Autodesk Inventor part; units mm, degrees
ref_plane "YZ Plane" through (0, 0, 0) normal (1, 0, 0) x (0, 1, 0)
ref_plane "XZ Plane" through (0, 0, 0) normal (0, 1, 0) x (-1, 0, 0)
ref_plane "XY Plane" through (0, 0, 0) normal (0, 0, 1) x (1, 0, 0)
sketch "スケッチ1" plane through (0, 0, 0) normal (1, 0, 0) x (0, 1, 0)
  line L0 (0, 0) -> (0, -38)
  line L1 (0, -38) -> (-10, -38)
  line L2 (-10, -38) -> (-10, 0)
  line L3 (-10, 0) -> (0, 0)
  dimension "d0" = 38
  dimension "d2" = 10
extrude "プレート1" add sketch "スケッチ1" along normal blind 2
sketch "スケッチ14" plane through (-2, 2, -38) normal (0, 1, 0) x (-1, 0, 0)
  line L0 (0, 38) -> (0, 0)
  line L1 (0, 0) -> (8, 0)
  line L2 (8, 0) -> (8, 38)
  line L3 (8, 38) -> (0, 38)
edge flange "フランジ1" height 12 angle 90 thickness 2 bend radius 2 thickness toward (0, 1, 0) relief tear relief width 2 relief depth 1 edges at (0, 0, -19) wall of the first edge with corners at (-2, 2, 0) (-2, 2, -38) (-10, 2, -38) (-10, 2, 0)
bend "曲げ26"
corner "コーナー1"
sketch "スケッチ15" plane through (-2, -12, 0) normal (0, -1, 0) x (1, 0, 0)
  line L0 (0, -38) -> (0, 0)
  line L1 (0, 0) -> (-8, 0)
  line L2 (-8, 0) -> (-8, -38)
  line L3 (-8, -38) -> (0, -38)
edge flange "フランジ2" height 12 angle 90 thickness 2 bend radius 2 thickness toward (0, -1, 0) relief tear relief width 2 relief depth 1 edges at (0, -10, -19) wall of the first edge with corners at (-2, -12, -38) (-2, -12, 0) (-10, -12, 0) (-10, -12, -38)
bend "曲げ27"
corner "コーナー2"
sketch "スケッチ16" plane through (-10, 4, 0) normal (0, 1, 0) x (1, 0, 0)
  line L0 (5.5, 4) -> (5.5, 34)
  arc A0 (5.5, 34) -> (2.5, 34) centre (4, 34) ccw
  line L1 (2.5, 34) -> (2.5, 4)
  arc A1 (2.5, 4) -> (5.5, 4) centre (4, 4) ccw
  line L2 (0, 38) -> (8, 38)
  line L3 (8, 0) -> (0, 0)
  point P0 (10, 0)
  point P1 (4, 38)
  dimension "d192" = 1.5
  dimension "d193" = 4
  dimension "d194" = 4
extrude "押し出し1" cut sketch "スケッチ16" against normal blind 10
sketch "スケッチ17" plane through (-10, -12, 0) normal (0, 1, 0) x (1, 0, 0)
  line L0 (0, 0) -> (8, 0)
  line L1 (0, 38) -> (8, 38)
  point P0 (10, 0)
  point P1 (4, 5)
  point P2 (4, 33)
  point P3 (4, 0)
  point P4 (4, 38)
  dimension "d197" = 5
  dimension "d198" = 5
hole "穴1" at (-6, -12, -5) at (-6, -12, -33) direction (0, -1, 0) diameter 3 end through all
equation "\"d204\" = Thickness"
equation "\"d3\" = Thickness"
equation "\"d172\" = BendReliefWidth"
equation "\"d173\" = BendReliefDepth"
equation "\"d174\" = MinimumRemnant"
equation "\"d175\" = TransitionRadius"
equation "\"d178\" = BendRadius"
equation "\"d179\" = CornerReliefSize"
equation "\"d180\" = GapSize"
equation "\"d181\" = JacobiRadiusSize"
equation "\"d182\" = BendReliefWidth"
equation "\"d183\" = BendReliefDepth"
equation "\"d184\" = MinimumRemnant"
equation "\"d185\" = TransitionRadius"
equation "\"d188\" = BendRadius"
equation "\"d189\" = CornerReliefSize"
equation "\"d190\" = GapSize"
equation "\"d191\" = JacobiRadiusSize"
equation "\"BendRadius\" = Thickness"
equation "\"BendReliefWidth\" = Thickness"
equation "\"BendReliefDepth\" = 0.5 * Thickness"
equation "\"CornerReliefSize\" = 4 * Thickness"
equation "\"MinimumRemnant\" = 2 * Thickness"
equation "\"TransitionRadius\" = BendRadius"
equation "\"JacobiRadiusSize\" = BendRadius"
equation "\"GapSize\" = Thickness"
properties part number "frame_front" material "アルミニウム 6061"
Geometry check sheet. Reference: the model listing, model coordinates, mm. A direction names the side the tool comes from. Round coordinates to 2 decimals unless told otherwise and drop trailing zeros. Order: outer loops, then holes, each group sorted by start corner. A loop starts at its lowest first (then second) coordinate and runs counter-clockwise, first axis right, second up. Notation, with made-up numbers: M -25,72 L -5,72 A17 ccw -5,92 Z; hole C 54,17 d5. An arc over 180 degrees is marked long. Answer in a Markdown table with one row per item.
(1) Draft check along Y on faces 4 (the face through (0.4, -5.7, 0)), 5 (the face through (0.797, -12.859, -18.734)), 6 (the face through (-8, 4, -19)), 7 (the face through (-0.6, 1.43, -19.27)). Enter one of: released by +Y, released by -Y, zero draft, split by the parting line, or undercut.
Responses:
| item | result |
|---|---|
| face 4 | zero draft |
| face 5 | released by -Y |
| face 6 | released by +Y |
| face 7 | undercut |
(2) Sectioned sample at B-B, the plane x = -6. Record the cut outline in (y, z), and give its area (3 significant figures).
Responses:
| item | result |
|---|---|
| outline | M -14,-38 L -12,-38 L -12,-34.5 L -14,-34.5 Z; M -14,-31.5 L -12,-31.5 L -12,-6.5 L -14,-6.5 Z; M -14,-3.5 L -12,-3.5 L -12,0 L -14,0 Z; M 2,-38 L 4,-38 L 4,-35.5 L 2,-35.5 Z; M 2,-2.5 L 4,-2.5 L 4,0 L 2,0 Z |
| area | 74.0 mm² |
(3) Sectioned sample at A-A, the plane x = -2.5. Record the cut outline in (y, z), and give its area (3 significant figures).
Responses:
| item | result |
|---|---|
| outline | M -14,-38 L -12,-38 L -12,0 L -14,0 Z; M 2,-38 L 4,-38 L 4,0 L 2,0 Z |
| area | 152 mm² |
(4) Sectioned sample at C-C, the plane z = -10. Record the cut outline in (x, y), and give its area (3 significant figures).
Responses:
| item | result |
|---|---|
| outline | M -10,-14 L -2,-14 A4 ccw 2,-10 L 2,0 A4 ccw -2,4 L -4.5,4 L -4.5,2 L -2,2 A2 cw 0,0 L 0,-10 A2 cw -2,-12 L -10,-12 Z; M -10,2 L -7.5,2 L -7.5,4 L -10,4 Z |
| area | 64.8 mm² |
(5) Go/stop test with flat-tipped pins: P1, Ø2.5, axis at x = -6, z = -33, coming from the -Y side; P2, Ø8, axis at y = -7, z = -18.5, coming from the -X side; P3, Ø1.6, axis at y = 3.5, z = -13.5, coming from the +X side; P4, Ø8, axis at y = -6, z = -21, coming from the -X side. Record where each tip stops, or that it passes through.
Responses:
| item | result |
|---|---|
| P1 | passes through |
| P2 | stops at x = -0.27 |
| P3 | stops at x = 0.95 |
| P4 | stops at x = 0 |
(6) Sectioned sample at D-D, the plane z = -5.5. Record the cut outline in (x, y).
Responses:
| item | result |
|---|---|
| outline | M -10,-14 L -7.41,-14 L -7.41,-12 L -10,-12 Z; M -10,2 L -7.5,2 L -7.5,4 L -10,4 Z; M -4.59,-14 L -2,-14 A4 ccw 2,-10 L 2,0 A4 ccw -2,4 L -4.5,4 L -4.5,2 L -2,2 A2 cw 0,0 L 0,-10 A2 cw -2,-12 L -4.59,-12 Z |
(7) Tool access check on faces 1 (the face through (-7.5, 3, -19)), 2 (the face through (-5.1, -13, -34.2)), 3 (the face through (-6, -12, -19)). Record the directions out of +Z, -Z, +X, -X, +Y, -Y that give a thin tool (end or side, any length) a straight path to the whole face; none if there is none.
Responses:
| item | result |
|---|---|
| face 1 | +Y |
| face 2 | +Y, -Y |
| face 3 | +Z, -Z, -X |
(8) Scan lines: probe 1 along Z at (x, y) = (-6, -13.1); probe 2 along Y at (x, z) = (-8, -34); probe 3 along X at (y, z) = (-9.25, -5.5). Record each from-to range of solid material in increasing order. Write a range as from..to.
Responses:
| item | result |
|---|---|
| probe 1 | z = -38..-34.5, -31.5..-6.5, -3.5..0 |
| probe 2 | y = -14..-12, 2..4 |
| probe 3 | x = 0..2 |
